Read the model definition and answer for the solid it produces. Units are mm, in the model's axes. A direction names the side the tool comes from. Coordinates: 2 decimals unless noted, no trailing zeros. Write each loop counter-clockwise with the first axis right and the second up, starting at its lowest first coordinate (ties: lowest second). Pieces come first, ordered by that corner, then holes.
(1) Section B-B on y = 57 is taken. Write down the section's boundary in (x, z).
(2) Section A-A on x = 3.5 is taken. Write down the section's boundary in (y, z).
(3) Which of the six approach directions +Z, -Z, +X, -X, +Y, -Y give full straight-line access (tool end or side, diameter ignored) to faces 1 (the cylindrical face through (-15.292, 1.972, 4.173)), 2 (the cylindrical face through (-30, 19, 24)), 3 (the flat face through (-12, 4, -13))?
(4) Find the intervals of material crossed by probe 1 along X at (y, z) = (1.25, 23.5); probe 2 along Z at (x, y) = (27, 2); probe 3 along Z at (x, y) = (3, 3), in increasing order.
(5) Given pin 1 (1.5 mm diameter, centred on x = -11, z = 21.5, fed in from +Y); pin 2 (4.5 mm diameter, centred on x = -30.5, z = 15, fed in from -Y); pin 3 (3 mm diameter, centred on y = 13.5, z = 10, fed in from +X), each flat-ended and moving along its own axis, determine where each tip first touches the part or whether it passes through.
(6) Section C-C on x = -20 is taken. Write down the section's boundary in (y, z).
(7) Section D-D on z = -8.5 is taken. Write down the section's boundary in (x, y).
(8) The mould has two halves that part along X. Classify faces 4 (the cylindrical face through (-22, 2, -25)), 5 (the flat face through (-28, 34, 0)), 6 (the flat face through (-32, 32, 0)), 7 (the flat face through (-30, 16.5, 17)): +X half, -X half, draft (parallel to the pull), parting line (faces both ways), or undercut.
from build123d import *

# Parameters (mm, degrees)
SKETCH1_W                = 64
SKETCH1_H                = 57
BOSS_EXTRUDE1_DEPTH      = 4
SKETCH2_W                = 4
SKETCH2_H                = 57
BOSS_EXTRUDE2_DEPTH      = 60
SKETCH3_R                = 19.25
CUT_EXTRUDE1_DEPTH       = 60
F_5_0_5_DIAMETER_HOLE1_D = 5
CUT_EXTRUDE2_DEPTH       = 60


with BuildPart() as part:
    # Sketch1 → Boss-Extrude1 (new body)
    with BuildSketch(Plane(origin=(0, 0, 0), x_dir=(1, 0, 0), z_dir=(0, 1, 0))):
        Rectangle(SKETCH1_W, SKETCH1_H)
    extrude(amount=BOSS_EXTRUDE1_DEPTH)

    # Sketch2 → Boss-Extrude2 (add)
    with BuildSketch(Plane(origin=(0, 4, 0), x_dir=(1, 0, 0), z_dir=(0, 1, 0))):
        with Locations((-30, 0)):
            Rectangle(SKETCH2_W, SKETCH2_H)
    extrude(amount=BOSS_EXTRUDE2_DEPTH)

    # Sketch3 → Cut-Extrude1 (cut)
    with BuildSketch(Plane.XZ):
        with Locations(Location((3.5, 0, 0), (0, 0, 270))):
            Circle(SKETCH3_R)
    extrude(amount=-CUT_EXTRUDE1_DEPTH, mode=Mode.SUBTRACT)

    # Ø5.0 (5) Diameter Hole1 (through all)
    with Locations(Plane(origin=(0, 0, 0), x_dir=(-1, 0, 0), z_dir=(0, -1, 0))):
        with Locations((-27, -23.5), (-27, 23.5), (20, 23.5), (20, -23.5)):
            Hole(F_5_0_5_DIAMETER_HOLE1_D / 2)

    # Sketch6 → Cut-Extrude2 (cut)
    with BuildSketch(Plane.ZY.offset(32)):
        with BuildLine():
            Line((-21.5, 16.5), (-12.5, 16.5))
            ThreePointArc((-12.5, 16.5), (-10, 19), (-12.5, 21.5))
            Line((-12.5, 21.5), (-21.5, 21.5))
            ThreePointArc((-21.5, 21.5), (-24, 19), (-21.5, 16.5))
        make_face()
        with BuildLine():
            Line((12.5, 16.5), (21.5, 16.5))
            ThreePointArc((21.5, 16.5), (24, 19), (21.5, 21.5))
            Line((21.5, 21.5), (12.5, 21.5))
            ThreePointArc((12.5, 21.5), (10, 19), (12.5, 16.5))
        make_face()
        with BuildLine():
            Line((-21.5, 54.5), (-12.5, 54.5))
            ThreePointArc((-12.5, 54.5), (-10, 57), (-12.5, 59.5))
            Line((-12.5, 59.5), (-21.5, 59.5))
            ThreePointArc((-21.5, 59.5), (-24, 57), (-21.5, 54.5))
        make_face()
        with BuildLine():
            Line((12.5, 54.5), (21.5, 54.5))
            ThreePointArc((21.5, 54.5), (24, 57), (21.5, 59.5))
            Line((21.5, 59.5), (12.5, 59.5))
            ThreePointArc((12.5, 59.5), (10, 57), (12.5, 54.5))
        make_face()
    extrude(amount=-CUT_EXTRUDE2_DEPTH, mode=Mode.SUBTRACT)


solid = part.part
Response:
1. outline: (-32, -28.5) - (-28, -28.5) - (-28, -24) - (-32, -24) - close; (-32, -10) - (-28, -10) - (-28, 10) - (-32, 10) - close; (-32, 24) - (-28, 24) - (-28, 28.5) - (-32, 28.5) - close
2. outline: (0, -28.5) - (4, -28.5) - (4, -19.25) - (0, -19.25) - close; (0, 19.25) - (4, 19.25) - (4, 28.5) - (0, 28.5) - close
3. face 1: +Y, -Y
3. face 2: +X, -X
3. face 3: +Z, -Z, +X, +Y
4. probe 1: x = -32 to -22.5, -17.5 to 24.5, 29.5 to 32
4. probe 2: z = -28.5 to -26, -21 to 21, 26 to 28.5
4. probe 3: z = -28.5 to -19.24, 19.24 to 28.5
5. pin 1: stops at y = 4
5. pin 2: stops at y = 0
5. pin 3: stops at x = -28
6. outline: (0, -28.5) - (4, -28.5) - (4, -26) - (0, -26) - close; (0, -21) - (4, -21) - (4, 21) - (0, 21) - close; (0, 26) - (4, 26) - (4, 28.5) - (0, 28.5) - close
7. outline: (-32, 0) - (-13.77, 0) - (-13.77, 4) - (-28, 4) - (-28, 64) - (-32, 64) - close; (20.77, 0) - (32, 0) - (32, 4) - (20.77, 4) - close
8. face 4: undercut
8. face 5: +X half
8. face 6: -X half
8. face 7: draft
